Verification items for the finished model (mm, model axes). A direction names the side the tool comes from. Coordinates: 2 decimals unless noted, no trailing zeros. Write each loop counter-clockwise with the first axis right and the second up, starting at its lowest first coordinate (ties: lowest second). Pieces come first, ordered by that corner, then holes. Notation, with made-up numbers: (1, 21.5) - (22, 21.5) arc R32 cw to (22, 56.5) - close; hole circle Ø3 at (0.5, 89). An arc over 180 degrees is marked (long way). Use one line per item in the form item = value. Start each with the question number.
(1) Gauge pin test, flat ends, axial feed: pin 1 Ø3 at (x, z) = (28, 5) entering from -Y; pin 2 Ø3 at (x, y) = (1, -48.5) entering from -Z. Record the tip position at first contact, or that the pin passes through.
(2) Mould release check, pull along Y, two halves, no side actions. Record for faces 1 (the cylindrical face through (20.632, 50.255, 3.219)), 2 (the cylindrical face through (30.813, -33.925, 1.761)): released by +Y, released by -Y, zero draft, split by the parting line, or undercut.
(3) Sectioned sample at B-B (y = -50). Record the cut outline in (x, z), and give its area (3 significant figures).
(4) Material ranges on line 1 (X direction, y = -11.5, z = 5); line 2 (X direction, y = 22, z = 4.5); line 3 (Y direction, x = -47, z = 1.75), recorded low to high. Write a range as [from, to].
(5) Tool access check on faces 3 (the flat face through (6.6, -50.13, 3.22)), 4 (the cylindrical face through (48.826, 24.35, 1.761)). Record the directions out of +Z, -Z, +X, -X, +Y, -Y that give a thin tool (end or side, any length) a straight path to the whole face; none if there is none.
(6) Sectioned sample at A-A (x = -16.5). Record the cut outline in (y, z).
(7) Sectioned sample at C-C (x = 0). Count the separate pieces of the cut face and the enclosed holes in it, and give its area (3 significant figures).
from build123d import *

# Parameters (mm, degrees)
SKETCH1_R                = 60.5
SKETCH1_R_2              = 1.89865
SKETCH1_R_3              = 1.9939
SKETCH1_R_4              = 8
BOSS_EXTRUDE1_DEPTH      = 6.35
CUT_EXTRUDE1_DEPTH       = 7.35
FILLET1_R                = 2
CIRPATTERN1_COUNT        = 8
FILLET1_OF_CIRPATTERN1_R = 2
CUT_EXTRUDE2_DEPTH       = 7.35
FILLET2_R                = 2
CIRPATTERN3_COUNT        = 8
FILLET2_OF_CIRPATTERN3_R = 2
SKETCH4_R                = 4.7625
SKETCH4_R_2              = 1.89865
CUT_EXTRUDE3_DEPTH       = 3.571875


with BuildPart() as part:
    # Sketch1 → Boss-Extrude1 (new body)
    with BuildSketch(Plane.XY):
        Circle(SKETCH1_R)
        with Locations((45.315389352, 21.130913087)):
            Circle(SKETCH1_R_2, mode=Mode.SUBTRACT)
        with Locations((49.978847504, 1.454235937)):
            Circle(SKETCH1_R_3, mode=Mode.SUBTRACT)
        Circle(SKETCH1_R_4, mode=Mode.SUBTRACT)
        with Locations((46.467376211, -18.460307366)):
            Circle(SKETCH1_R_3, mode=Mode.SUBTRACT)
        with Locations((0, -16.5)):
            Circle(SKETCH1_R_3, mode=Mode.SUBTRACT)
        with Locations((0, -50)):
            Circle(SKETCH1_R_2, mode=Mode.SUBTRACT)
        with Locations((-16.5, 0)):
            Circle(SKETCH1_R_3, mode=Mode.SUBTRACT)
        with Locations((-11.66726189, -11.66726189)):
            Circle(SKETCH1_R_2, mode=Mode.SUBTRACT)
        with Locations((0, 16.5)):
            Circle(SKETCH1_R_3, mode=Mode.SUBTRACT)
        with Locations((-11.66726189, 11.66726189)):
            Circle(SKETCH1_R_2, mode=Mode.SUBTRACT)
        with Locations((11.66726189, 11.66726189)):
            Circle(SKETCH1_R_2, mode=Mode.SUBTRACT)
        with Locations((-35.355339059, -35.355339059)):
            Circle(SKETCH1_R_2, mode=Mode.SUBTRACT)
        with Locations((-50, 0)):
            Circle(SKETCH1_R_2, mode=Mode.SUBTRACT)
        with Locations((-35.355339059, 35.355339059)):
            Circle(SKETCH1_R_2, mode=Mode.SUBTRACT)
        with Locations((0, 50)):
            Circle(SKETCH1_R_2, mode=Mode.SUBTRACT)
        with Locations((35.355339059, -35.355339059)):
            Circle(SKETCH1_R_2, mode=Mode.SUBTRACT)
    extrude(amount=BOSS_EXTRUDE1_DEPTH)

    # Sketch2 → Cut-Extrude1 (cut, through all)
    with BuildSketch(Plane.XY.offset(6.35)):
        with BuildLine():
            Line((-22.071405131, 5.914015181), (-42.162662318, 11.297451319))
            ThreePointArc((-42.162662318, 11.297451319), (-43.65, 0), (-42.162662318, -11.297451319))
            Line((-42.162662318, -11.297451319), (-22.071405131, -5.914015181))
            ThreePointArc((-22.071405131, -5.914015181), (-22.85, 0), (-22.071405131, 5.914015181))
        make_face()
    cut_extrude1 = extrude(amount=-CUT_EXTRUDE1_DEPTH, mode=Mode.SUBTRACT)

    # Fillet1
    fillet1_edges = [part.edges().sort_by_distance(p)[0] for p in [
        (-42.162662318, -11.297451319, 3.175),
        (-42.162662318, 11.297451319, 3.175),
        (-22.071405131, 5.914015181, 3.175),
        (-22.071405131, -5.914015181, 3.175),
    ]]
    fillet(fillet1_edges, radius=FILLET1_R)

    # CirPattern1: Cut-Extrude1 ×8 about axis, 3 skipped
    cirpattern1_axis = Axis((0, 0, 0), (0, 0, -1))
    add([cut_extrude1.rotate(cirpattern1_axis, i * 360 / CIRPATTERN1_COUNT) for i in range(1, CIRPATTERN1_COUNT) if i not in (3, 4, 5)], mode=Mode.SUBTRACT)

    # Fillet1 of CirPattern1
    fillet1_of_cirpattern1_edges = [part.edges().sort_by_distance(p)[0] for p in [
        (-37.802008875, 21.825, 3.175),
        (-21.825, 37.802008875, 3.175),
        (-11.425, 19.788680476, 3.175),
        (-19.788680476, 11.425, 3.175),
        (-11.297451319, 42.162662318, 3.175),
        (11.297451319, 42.162662318, 3.175),
        (5.914015181, 22.071405131, 3.175),
        (-5.914015181, 22.071405131, 3.175),
        (11.297451319, -42.162662318, 3.175),
        (-11.297451319, -42.162662318, 3.175),
        (-5.914015181, -22.071405131, 3.175),
        (5.914015181, -22.071405131, 3.175),
        (-21.825, -37.802008875, 3.175),
        (-37.802008875, -21.825, 3.175),
        (-19.788680476, -11.425, 3.175),
        (-11.425, -19.788680476, 3.175),
    ]]
    fillet(fillet1_of_cirpattern1_edges, radius=FILLET1_OF_CIRPATTERN1_R)

    # Sketch3 → Cut-Extrude2 (cut, through all)
    with BuildSketch(Plane.XY.offset(6.35)):
        with BuildLine():
            Line((-43.098920211, 33.070964631), (-37.148770159, 28.505253913))
            ThreePointArc((-37.148770159, 28.505253913), (-43.26065911, 17.91915172), (-46.424405634, 6.111888951))
            Line((-46.424405634, 6.111888951), (-53.860242094, 7.090835392))
            ThreePointArc((-53.860242094, 7.090835392), (-50.189755604, 20.789277463), (-43.098920211, 33.070964631))
        make_face()
    cut_extrude2 = extrude(amount=-CUT_EXTRUDE2_DEPTH, mode=Mode.SUBTRACT)

    # Fillet2
    fillet2_edges = [part.edges().sort_by_distance(p)[0] for p in [
        (-53.860242094, 7.090835392, 3.175),
        (-43.098920211, 33.070964631, 3.175),
        (-37.148770159, 28.505253913, 3.175),
        (-46.424405634, 6.111888951, 3.175),
    ]]
    fillet(fillet2_edges, radius=FILLET2_R)

    # CirPattern3: Cut-Extrude2 ×8 about axis, 2 skipped
    cirpattern3_axis = Axis((0, 0, 0), (0, 0, -1))
    add([cut_extrude2.rotate(cirpattern3_axis, i * 360 / CIRPATTERN3_COUNT) for i in range(1, CIRPATTERN3_COUNT) if i not in (3, 4)], mode=Mode.SUBTRACT)

    # Fillet2 of CirPattern3
    fillet2_of_cirpattern3_edges = [part.edges().sort_by_distance(p)[0] for p in [
        (-33.070964631, 43.098920211, 3.175),
        (-7.090835392, 53.860242094, 3.175),
        (-6.111888951, 46.424405634, 3.175),
        (-28.505253913, 37.148770159, 3.175),
        (7.090835392, 53.860242094, 3.175),
        (33.070964631, 43.098920211, 3.175),
        (28.505253913, 37.148770159, 3.175),
        (6.111888951, 46.424405634, 3.175),
        (33.070964631, -43.098920211, 3.175),
        (7.090835392, -53.860242094, 3.175),
        (6.111888951, -46.424405634, 3.175),
        (28.505253913, -37.148770159, 3.175),
        (-7.090835392, -53.860242094, 3.175),
        (-33.070964631, -43.098920211, 3.175),
        (-28.505253913, -37.148770159, 3.175),
        (-6.111888951, -46.424405634, 3.175),
        (-43.098920211, -33.070964631, 3.175),
        (-53.860242094, -7.090835392, 3.175),
        (-46.424405634, -6.111888951, 3.175),
        (-37.148770159, -28.505253913, 3.175),
    ]]
    fillet(fillet2_of_cirpattern3_edges, radius=FILLET2_OF_CIRPATTERN3_R)

    # Sketch4 → Cut-Extrude3 (cut)
    with BuildSketch(Plane(origin=(0, 0, 0), x_dir=(-1, 0, 0), z_dir=(0, 0, -1))):
        with Locations((0, 50)):
            Circle(SKETCH4_R)
        with Locations((0, 50)):
            Circle(SKETCH4_R_2, mode=Mode.SUBTRACT)
        with Locations((35.355339059, 35.355339059)):
            Circle(SKETCH4_R)
        with Locations((35.355339059, 35.355339059)):
            Circle(SKETCH4_R_2, mode=Mode.SUBTRACT)
        with Locations((50, 0)):
            Circle(SKETCH4_R)
        with Locations((50, 0)):
            Circle(SKETCH4_R_2, mode=Mode.SUBTRACT)
        with Locations((35.355339059, -35.355339059)):
            Circle(SKETCH4_R)
        with Locations((35.355339059, -35.355339059)):
            Circle(SKETCH4_R_2, mode=Mode.SUBTRACT)
        with Locations((0, -50)):
            Circle(SKETCH4_R)
        with Locations((0, -50)):
            Circle(SKETCH4_R_2, mode=Mode.SUBTRACT)
        with Locations((-35.355339059, -35.355339059)):
            Circle(SKETCH4_R)
        with Locations((-35.355339059, -35.355339059)):
            Circle(SKETCH4_R_2, mode=Mode.SUBTRACT)
        with Locations((-45.315389352, 21.130913087)):
            Circle(SKETCH4_R)
        with Locations((-45.315389352, 21.130913087)):
            Circle(SKETCH4_R_2, mode=Mode.SUBTRACT)
    extrude(amount=-CUT_EXTRUDE3_DEPTH, mode=Mode.SUBTRACT)


solid = part.part
Answers below:
q1.pin_1 = -54.39
q1.pin_2 = 3.57
q2.face_1 = undercut
q2.face_2 = undercut
q3.outline = (-34.06, 0) - (-21.24, 0) - (-21.24, 6.35) - (-34.06, 6.35) - close; (-6.58, 0) - (-4.76, 0) - (-4.76, 3.57) - (-1.9, 3.57) - (-1.9, 6.35) - (-6.58, 6.35) - close; (1.9, 3.57) - (4.76, 3.57) - (4.76, 0) - (6.58, 0) - (6.58, 6.35) - (1.9, 6.35) - close; (21.24, 0) - (34.06, 0) - (34.06, 6.35) - (21.24, 6.35) - close
q3.area = 202 mm2
q4.line_1 = [-59.4, -53.09], [-45.39, -13.56], [-9.78, 59.4]
q4.line_2 = [-56.36, -49.67], [-41.33, -36.96], [-12.7, 43.63], [47, 56.36]
q4.line_3 = [-38.1, -27.24], [-6.68, -3.7], [3.7, 6.68], [27.24, 38.1]
q5.face_3 = +Z, -Z
q5.face_4 = -Z
q6.outline = (-58.21, 0) - (-51.76, 0) - (-51.76, 6.35) - (-58.21, 6.35) - close; (-43.82, 0) - (-28.58, 0) - (-28.58, 6.35) - (-43.82, 6.35) - close; (-15.81, 0) - (-1.99, 0) - (-1.99, 6.35) - (-15.81, 6.35) - close; (1.99, 0) - (15.81, 0) - (15.81, 6.35) - (1.99, 6.35) - close; (28.58, 0) - (43.82, 0) - (43.82, 6.35) - (28.58, 6.35) - close; (51.76, 0) - (58.21, 0) - (58.21, 6.35) - (51.76, 6.35) - close
q7.separate_pieces = 8
q7.enclosed_holes = 0
q7.area = 263 mm2
